Source: CAD feature listing. Evaluate the final solid. Frame: model axes, mm. A direction names the side the tool comes from. Give positions to 0.01 mm unless a question says otherwise; leave off trailing zeros. Loops run counter-clockwise (first coordinate to the right, second up) from the corner with the lowest first, then second, coordinate; pieces in that order, holes last.
```python
from build123d import *

# Parameters (mm, degrees)
F1_DEPTH = 15
F3_DEPTH = 43.9597531212
F5_D     = 4
F6_R     = 10
F7_SIZE  = 5


with BuildPart() as f1:
    # F0 (on Front) → F1 (new body, symmetric)
    with BuildSketch(Plane.XZ):
        Polygon((50, 0), (0, 0), (0, -8.8), (45.8964926082, -8.8), (75.3981893849, -43.9587531212), (82.1393804843, -38.3022221559), align=None)
    extrude(amount=F1_DEPTH, both=True)

    # F2 (on face) → F3 (cut, through all)
    with BuildSketch(Plane.XY):
        with BuildLine():
            ThreePointArc((15.8875472844, 3), (12.8875472844, 0), (15.8875472844, -3))
            Line((15.8875472844, -3), (35.4375839233, -3))
            ThreePointArc((35.4375839233, -3), (38.4375839233, 0), (35.4375839233, 3))
            Line((35.4375839233, 3), (15.8875472844, 3))
        make_face()
    extrude(amount=-F3_DEPTH, mode=Mode.SUBTRACT)

    # F5 (through all)
    with Locations(Plane(origin=(29.3412044417, 0, 24.6201938253), x_dir=(0, 1, 0), z_dir=(0.7660444431, 0, 0.6427876097))):
        with Locations((0, -47.1393804843), (0, -67.1393804843)):
            Hole(F5_D / 2)

    # F6
    f6_edges = [f1.edges().sort_by_distance(p)[0] for p in [
        (78.768785, -15, -41.130488),
        (78.768785, 15, -41.130488),
    ]]
    fillet(f6_edges, radius=F6_R)

    # F7
    f7_edges = [f1.edges().sort_by_distance(p)[0] for p in [
        (0, -15, -4.4),
        (0, 15, -4.4),
    ]]
    chamfer(f7_edges, length=F7_SIZE)


solid = f1.part
```
(1) Mould query, pull axis Z, two halves, no side actions, for faces 3 (the flat face through (23, -4, -8.8)), 4 (the cylindrical face through (55.14, -1.08, -13.07)), 5 (the flat face through (42.81, 15, -8.65)). Classes: pulls with the +Z half, pulls with the -Z half, needs draft (parallel to the pull), parting line crosses it, or undercut.
A:
face 3: pulls with the -Z half
face 4: undercut
face 5: needs draft
(2) Reachability of faces 1 (the flat face through (26, 3, -4)), 2 (the flat face through (3, -13, -4)) from +Z, -Z, +X, -X, +Y, -Y: full face, straight path, thin tool, end or side. Return the list, or none.
A:
face 1: +Z, -Z
face 2: +Z, -Z, -X, -Y
(3) Section A-A, the plane x = 32. Return the cut outline in (y, z), then the cut area to 3 significant figures.
A:
outline: (-15, -8.8) - (-3, -8.8) - (-3, 0) - (-15, 0) - close; (3, -8.8) - (15, -8.8) - (15, 0) - (3, 0) - close
area: 211 mm2
(4) Section B-B, the plane y = 0. Return the cut outline in (x, z).
A:
outline: (0, -8.8) - (12.89, -8.8) - (12.89, 0) - (0, 0) - close; (38.44, -8.8) - (45.9, -8.8) - (51.62, -15.62) - (58.36, -9.96) - (50, 0) - (38.44, 0) - close; (54.19, -18.68) - (64.47, -30.94) - (71.21, -25.28) - (60.93, -13.02) - close; (67.04, -34) - (75.4, -43.96) - (82.14, -38.3) - (73.78, -28.34) - close
(5) Section C-C, the plane x = 11. Return the cut outline in (y, z).
A:
outline: (-15, -8.8) - (15, -8.8) - (15, 0) - (-15, 0) - close
(6) Ray query, line 1 along Y through (x, z) = (17.5, -6.5); line 2 along Z through (x, y) = (34, 9); line 3 along X through (y, z) = (2, -3). Return the intervals inside material, ascending.
A:
line 1: y = -15 to -3, 3 to 15
line 2: z = -8.8 to 0
line 3: x = 0 to 13.65, 37.67 to 52.52
(7) Section D-D, the plane z = -21. Return the cut outline in (x, y), then the cut area to 3 significant figures.
A:
outline: (56.13, -15) - (67.62, -15) - (67.62, 15) - (56.13, 15) - close
area: 345 mm2
(8) First-contact query: pin 1 (5 mm diameter, centred on y = 2.5, z = -34, fed in from +X); pin 2 (15 mm diameter, centred on x = 32, y = -6.5, fed in from -Z). Flat tips, straight axial feed; report the tip coordinate or a pass-through.
A:
pin 1: stops at x = 80.63
pin 2: stops at z = -8.8
